from build123d import *

# Parameters (mm, degrees)
F1_DEPTH      = 79.375
F4_DEPTH      = 19.05
F4_DEPTH_BACK = 19.05
F5_R          = 12.7
F7_W          = 9.525
F7_H          = 12.7
F8_DEPTH      = 3.175
F6_W          = 63.5
F6_H          = 10.3124
F6_R          = 4.9744809982
F9_DEPTH      = 3.9624
F10_SIZE2     = 1.818344
F10_SIZE      = 10.31239


# Not quite as in the source:
# - a fillet or chamfer is up to 0.001 mm smaller than in the source, because OpenCascade refuses the exact size


with BuildPart() as f1:
    # F0 (on Right) → F1 (new body)
    with BuildSketch(Plane.YZ):
        with BuildLine():
            Line((0, -9.525), (0, 0))
            Line((0, 0), (-57.15, 0))
            ThreePointArc((-57.15, 0), (-56.9498143774, -4.779240775), (-56.350659934, -9.525))
            Line((-56.350659934, -9.525), (-15.875, -9.525))
            Line((-15.875, -9.525), (0, -9.525))
        make_face()
        with BuildLine():
            ThreePointArc((-56.350659934, -9.525), (-56.9498143774, -4.779240775), (-57.15, 0))
            Line((-57.15, 0), (-69.85, 0))
            ThreePointArc((-69.85, 0), (-69.6866892703, -4.7736609169), (-69.1975207287, -9.525))
            Line((-69.1975207287, -9.525), (-56.350659934, -9.525))
        make_face()
        with BuildLine():
            Line((0, -57.15), (0, -9.525))
            Line((0, -9.525), (-15.875, -9.525))
            Line((-15.875, -9.525), (-15.875, -54.9008822789))
            ThreePointArc((-15.875, -54.9008822789), (-8.0167661111, -56.5849269781), (0, -57.15))
        make_face()
        with BuildLine():
            ThreePointArc((-69.1975207287, -9.525), (-69.6866892703, -4.7736609169), (-69.85, 0))
            Line((-69.85, 0), (-69.85, -9.525))
            Line((-69.85, -9.525), (-69.1975207287, -9.525))
        make_face()
        with BuildLine():
            ThreePointArc((-15.875, -54.9008822789), (-42.648319561, -38.042651572), (-56.350659934, -9.525))
            Line((-56.350659934, -9.525), (-69.1975207287, -9.525))
            ThreePointArc((-69.1975207287, -9.525), (-45.900442536, -52.6514185469), (0, -69.85))
            Line((0, -69.85), (0, -57.15))
            ThreePointArc((0, -57.15), (-8.0167661111, -56.5849269781), (-15.875, -54.9008822789))
        make_face()
    extrude(amount=-F1_DEPTH)

    # F3 (on offset) → F4 (cut, two sides)
    with BuildSketch(Plane.YZ.offset(-39.6875)) as f4_sk:
        with BuildLine():
            ThreePointArc((-21.853262225, -31.2096928874), (-33.7951127441, -17.5926221643), (-38.1, 0))
            Line((-38.1, 0), (-69.85, 0))
            Line((-69.85, 0), (-69.85, -9.525))
            Line((-69.85, -9.525), (-69.1975207287, -9.525))
            ThreePointArc((-69.1975207287, -9.525), (-59.6086170026, -36.4120210787), (-40.0643140791, -57.2177702936))
            Line((-40.0643140791, -57.2177702936), (-21.853262225, -31.2096928874))
        make_face()
        with BuildLine():
            ThreePointArc((-2.9503190018, -7.9502), (-3.1448391156, -6.5727258097), (-3.7131865837, -5.3029800181))
            Line((-3.7131865837, -5.3029800181), (-8.9719164583, -12.8132246066))
            ThreePointArc((-8.9719164583, -12.8132246066), (-4.7993720072, -11.8202337289), (-2.9503190018, -7.9502))
        make_face()
        with BuildLine():
            Line((-8.9719164583, -12.8132246066), (-3.7131865837, -5.3029800181))
            ThreePointArc((-3.7131865837, -5.3029800181), (-11.9996562789, -5.0969549164), (-8.9719164583, -12.8132246066))
        make_face()
    extrude(amount=-F4_DEPTH, mode=Mode.SUBTRACT)
    extrude(f4_sk.sketch, amount=F4_DEPTH_BACK, mode=Mode.SUBTRACT)

    # F5
    f5_edges = [f1.edges().sort_by_distance(p)[0] for p in [
        (-58.7375, -37.796331, -4.800764),
        (-58.7375, -36.422104, -52.016155),
        (-20.6375, -37.796331, -4.800764),
        (-20.6375, -36.422104, -52.016155),
    ]]
    fillet(f5_edges, radius=F5_R)

    # F7 (on face) → F8 (join)
    with BuildSketch(Plane(origin=(-79.375, 0, 0), x_dir=(0, -1, 0), z_dir=(-1, 0, 0))):
        with Locations((-4.7625, -63.5)):
            Rectangle(F7_W, F7_H)
    extrude(amount=-F8_DEPTH)

    # F6 (on face) → F9 (join)
    with BuildSketch(Plane.YZ):
        with Locations((-31.75, 5.1562)):
            Rectangle(F6_W, F6_H)
        Polygon((0, -15.875), (0, 0), (-63.5, 0), (-69.85, 0), (-69.85, -9.525), (-69.1975207287, -9.525), (-56.350659934, -9.525), (-15.875, -9.525), (-15.875, -15.875), align=None)
        with Locations((-7.9248, -7.9502)):
            Circle(F6_R, mode=Mode.SUBTRACT)
    extrude(amount=F9_DEPTH)

    # F10 (size 10.3124 and 1.8183543559 in the source; OpenCascade refuses exactly that, so slightly less here)
    f10_edges = [f1.edges().sort_by_distance(p)[0] for p in [
        (0, -31.75, 10.3124),
    ]]
    f10_side = f1.faces().sort_by_distance((0, -31.75, 5.1562))[0]
    chamfer(f10_edges, length=F10_SIZE, length2=F10_SIZE2, reference=f10_side)


solid = f1.part
Verification items for the finished model (mm, model axes). A direction names the side the tool comes from. Round coordinates to 2 decimals unless told otherwise and drop trailing zeros. Loops run counter-clockwise (first coordinate to the right, second up) from the corner with the lowest first, then second, coordinate; pieces in that order, holes last. Notation, with made-up numbers: (64, -39.75) - (115, -39.75) arc R18 ccw to (115, -30.75) - close; hole circle Ø4 at (46.25, 48.5). An arc over 180 degrees is marked (long way). Use a Markdown table: item, result. Add a question column.
1. Access from +Z, -Z, +X, -X, +Y, -Y to the whole of each face (thin tool, end or side, straight path). Record for faces 4 (the face through (-38, -15.875, -32)), 5 (the face through (-54.92, -38.92, -49.27)), 6 (the face through (-58.738, -8, -8)), 7 (the face through (0, -8, -8)).
2. Section check D-D, the plane y = -52. Give the number of separate pieces and of enclosed holes in the cut face, plus the area to 3 significant figures.
3. Section check B-B, the plane z = -21. Record the boundary of the cut face in (x, y) (1 decimal).
4. Section check A-A, the plane x = -14.5. Record the boundary of the cut face in (y, z) (3 decimals).
5. Release check for a two-part mould opening along Z. For faces 1 (the face through (-39.13, -31.57, -47.64)), 2 (the face through (-79.375, -12, -34)), 3 (the face through (3, -32, 10.312)) record: released by +Z, released by -Z, zero draft, split by the parting line, or undercut.
6. Gauge pin test, flat ends, axial feed: pin 1 (5 mm diameter, centred on y = -50.5, z = -19.5, fed in from -X); pin 2 (4 mm diameter, centred on x = -50, z = -56, fed in from +Y); pin 3 (10.5 mm diameter, centred on y = 3, z = -64.5, fed in from +X); pin 4 (16 mm diameter, centred on x = -53, y = -44.5, fed in from -Z). Record the tip position at first contact, or that the pin passes through.
7. Thickness scan on probe 1 along X at (y, z) = (-11.5, -7.5) (1 decimal); probe 2 along X at (y, z) = (-64, -6) (1 decimal); probe 3 along Y at (x, z) = (-60, -7). Record the ranges inside material, lowest first. Write a range as [from, to].
Checks:
| question | item | result |
|---|---|---|
| 1 | face 4 | +X, -X |
| 1 | face 5 | -Y |
| 1 | face 6 | none |
| 1 | face 7 | +X |
| 2 | separate pieces | 4 |
| 2 | enclosed holes | 0 |
| 2 | area | 1,410 mm^2 |
| 3 | outline | (-79.4, -66.6) - (-58.7, -66.6) - (-58.7, -53.2) - (-79.4, -53.2) - close; (-79.4, -15.9) - (0, -15.9) - (0, 0) - (-79.4, 0) - close; (-20.6, -66.6) - (0, -66.6) - (0, -53.2) - (-20.6, -53.2) - close |
| 4 | outline | (-69.85, -9.525) - (-69.198, -9.525) arc R69.85 ccw to (0, -69.85) - (0, 0) - (-69.85, 0) - close; hole (-56.351, -9.525) arc R57.15 ccw to (-15.875, -54.901) - (-15.875, -9.525) - close |
| 5 | face 1 | undercut |
| 5 | face 2 | zero draft |
| 5 | face 3 | released by +Z |
| 6 | pin 1 | passes through |
| 6 | pin 2 | stops at y = 0 |
| 6 | pin 3 | stops at x = 0 |
| 6 | pin 4 | stops at z = -59.55 |
| 7 | probe 1 | x = [-79.4, -58.7], [-20.6, 0] |
| 7 | probe 2 | x = [-79.4, -58.7], [-20.6, 4] |
| 7 | probe 3 | y = [-69.85, 0] |
